Read the model definition and answer for the solid it produces. Units are mm, in the model's axes. Coordinates: 2 decimals unless noted, no trailing zeros. Loops run counter-clockwise (first coordinate to the right, second up) from the corner with the lowest first, then second, coordinate; pieces in that order, holes last.
Q1. Straight lines are drawn through the part: line 1 (Z direction, x = 0, y = 1.75); line 2 (X direction, y = 3.05, z = 5.5); line 3 (Z direction, x = 2, y = 0.7). For each, find the intervals that lie inside material, in ascending order.
Q2. Section A-A (x = 0) is taken. Give the vertices of the cut face in (y, z) (3 decimals).
Q3. Section B-B (z = 0) is taken. Give the vertices of the cut face in (x, y) (3 decimals), then the cut area to 3 significant figures.
Q4. Flat-ended cylindrical pins translate along their axes: P1, Ø11, axis at x = 0, z = 0, coming from the +Y side; P2, Ø1, axis at y = 2.5, z = -20.5, coming from the +X side; P3, Ø1, axis at x = -45.5, y = 1.5, coming from the +Z side. Find the tip coordinate at first contact, or state that the pin passes through.
from build123d import *

# Parameters (mm, degrees)
SKETCH_1_W               = 70.7
SKETCH_1_H               = 4.9
CHAMFER_1_SIZE           = 1.645
CHAMFER_1_SIZE2          = 0.440776422
CHAMFER_2_SIZE           = 1.645
CHAMFER_2_SIZE2          = 0.440776422
SKETCH_2_R               = 6
CUT_EXTRUDE_3_DEPTH      = 1
CUT_EXTRUDE_3_DEPTH_BACK = 5.9


with BuildPart() as part:
    # Эскиз1 → Повернуть2 (revolve)
    with BuildSketch(Plane.XY):
        with Locations((35.35, 2.45)):
            Rectangle(SKETCH_1_W, SKETCH_1_H)
    revolve(axis=Axis((0, 4.9, 0), (0, -1, 0)))

    # Фаска1
    chamfer_1_edges = [part.edges().sort_by_distance(p)[0] for p in [
        (-70.7, 4.9, 0),
    ]]
    chamfer_1_side = [part.faces().sort_by_distance(p)[0] for p in [
        (0, 4.9, 0),
    ]]
    chamfer(chamfer_1_edges, length=CHAMFER_1_SIZE, length2=CHAMFER_1_SIZE2, reference=chamfer_1_side[0])

    # Фаска2
    chamfer_2_edges = [part.edges().sort_by_distance(p)[0] for p in [
        (-70.7, 0, 0),
    ]]
    chamfer_2_side = [part.faces().sort_by_distance(p)[0] for p in [
        (0, 0, 0),
    ]]
    chamfer(chamfer_2_edges, length=CHAMFER_2_SIZE, length2=CHAMFER_2_SIZE2, reference=chamfer_2_side[0])

    # Эскиз2 → Вырез-Вытянуть3 (cut, two sides)
    with BuildSketch(Plane(origin=(0, 0, 0), x_dir=(-1, 0, 0), z_dir=(0, -1, 0))) as cut_extrude_3_sk:
        Circle(SKETCH_2_R)
    extrude(amount=CUT_EXTRUDE_3_DEPTH, mode=Mode.SUBTRACT)
    extrude(cut_extrude_3_sk.sketch, amount=-CUT_EXTRUDE_3_DEPTH_BACK, mode=Mode.SUBTRACT)


solid = part.part
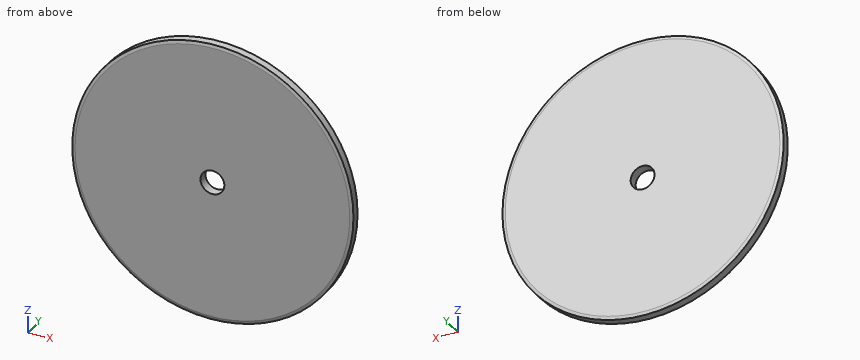
Numbers:
1. line 1: z = -70.7 to -6, 6 to 70.7
1. line 2: x = -70.49 to -2.4, 2.4 to 70.49
1. line 3: z = -70.67 to -5.66, 5.66 to 70.67
2. outline: (0, -69.055) - (0.441, -70.7) - (4.459, -70.7) - (4.9, -69.055) - (4.9, -6) - (0, -6) - close; (0, 6) - (4.9, 6) - (4.9, 69.055) - (4.459, 70.7) - (0.441, 70.7) - (0, 69.055) - close
3. outline: (-70.7, 0.441) - (-69.055, 0) - (-6, 0) - (-6, 4.9) - (-69.055, 4.9) - (-70.7, 4.459) - close; (6, 0) - (69.055, 0) - (70.7, 0.441) - (70.7, 4.459) - (69.055, 4.9) - (6, 4.9) - close
3. area: 633 mm2
4. P1: passes through
4. P2: stops at x = 67.81
4. P3: stops at z = 54.53
